For this review, take the finished solid that the model builds, in its own axes (mm). Face numbers are marked on the shaded views. A direction names the side the tool comes from. Round coordinates to 2 decimals unless told otherwise and drop trailing zeros. Loops run counter-clockwise (first coordinate to the right, second up) from the corner with the lowest first, then second, coordinate; pieces in that order, holes last. Notation, with made-up numbers: (75.25, 89.5) -> (132.25, 89.5) arc R17 ccw to (132.25, 99.5) -> close; hole circle Ø10 at (44, 28). An arc over 180 degrees is marked (long way). One line per question, with ' | ' between items. Start each with the question number.
1. Consider section D-D (x = 7). Write out the cut boundary in (y, z), and give its area (3 significant figures).
2. For the marked faces 4 and 5, list the 3-axis set-ups (+Z, -Z, +X, -X, +Y, -Y) from which the entire face can be reached by the end or side of a thin tool; tool diameter is ignored.
3. Consider section A-A (z = 0). Write out the cut boundary in (x, y), and give its area (3 significant figures).
4. Draft analysis for pull direction X (two halves, no side actions). For the marked faces 1, 2 and 3, state which applies: pulls with the +X half, pulls with the -X half, needs draft (parallel to the pull), parting line crosses it, or undercut.
5. Wall thickness on line 1 along Y through (x, z) = (14.5, -1.5); line 2 along Y through (x, z) = (12.5, 0); line 3 along X through (y, z) = (41, 0): over which ranges is each line inside the solid? List them lowest first.
6. For pin 1 Ø2 at (x, y) = (-0.5, 20) entering from -Z; pin 2 Ø10 at (x, y) = (-3, 26.5) entering from +Z; pin 3 Ø1.5 at (x, z) = (-3, -0.5) entering from +Y; pin 4 Ø8 at (y, z) = (12, 12) entering from -X, all flat-tipped, find the tip position at first contact; note any pin that passes through.
7. Consider section B-B (x = 0). Write out the cut boundary in (y, z), and give its area (4 significant figures).
8. Consider section C-C (y = 51). Write out the cut boundary in (x, z).
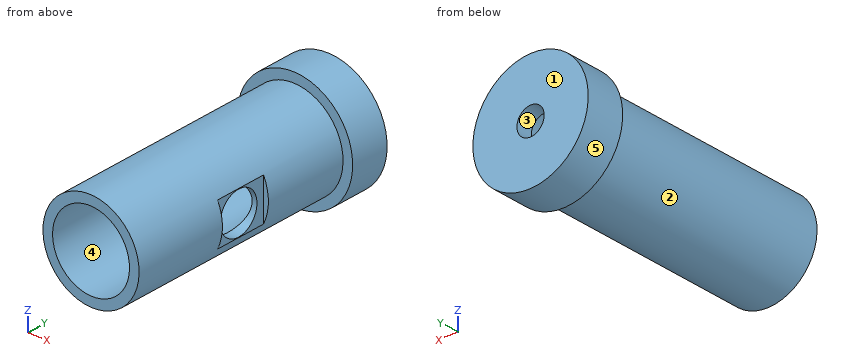
```python
from build123d import *

# Parameters (mm, degrees)
TAGLIO_ESTRUSIONE1_START = 15
SCHIZZO2_W               = 16
SCHIZZO2_H               = 16
TAGLIO_ESTRUSIONE1_DEPTH = 1.5
FORO_12_8_12_8_1_D       = 12.8
FORO_12_8_12_8_1_DEPTH   = 15.154492038
FORO_12_8_12_8_1_TIP     = 3.845507962


with BuildPart() as part:
    # Schizzo1 → Rivoluzione1 (revolve)
    with BuildSketch(Plane.XY, mode=Mode.PRIVATE) as rivoluzione1_sk:
        Polygon((-12, 0), (-15, 0), (-15, 71), (-18, 71), (-18, 83), (-4.25, 83), (-4.25, 78), (-12, 78), align=None)
    revolve(rivoluzione1_sk.sketch.rotate(Axis((0, 0, 0), (0, 1, 0)), 270), axis=Axis((0, 0, 0), (0, 1, 0)))

    # Schizzo2 → Taglio-Estrusione1 (cut)
    with BuildSketch(Plane(origin=(0, 0, 0), x_dir=(0, 0, -1), z_dir=(1, 0, 0)).offset(TAGLIO_ESTRUSIONE1_START)):
        with Locations((0, 37)):
            Rectangle(SCHIZZO2_W, SCHIZZO2_H)
    extrude(amount=-TAGLIO_ESTRUSIONE1_DEPTH, mode=Mode.SUBTRACT)

    # Foro Ø12.8 (12.8)-1
    with Locations(Plane(origin=(13.5, 0, 0), x_dir=(0, 0, -1), z_dir=(1, 0, 0))):
        with Locations((0, 36.304872912)):
            Hole(FORO_12_8_12_8_1_D / 2, depth=FORO_12_8_12_8_1_DEPTH)
            with Locations((0, 0, -(FORO_12_8_12_8_1_DEPTH + FORO_12_8_12_8_1_TIP / 2))):  # 118° drill point
                Cone(0, FORO_12_8_12_8_1_D / 2, FORO_12_8_12_8_1_TIP, mode=Mode.SUBTRACT)


solid = part.part
```
Answer block:
1) outline: (0, -13.27) -> (71, -13.27) -> (71, -16.58) -> (83, -16.58) -> (83, 16.58) -> (71, 16.58) -> (71, 13.27) -> (0, 13.27) -> (0, 9.75) -> (78, 9.75) -> (78, -9.75) -> (0, -9.75) -> close | area: 761 mm2
2) face 4: -Y | face 5: +Y, -Y
3) outline: (-18, 71) -> (-15, 71) -> (-15, 0) -> (-12, 0) -> (-12, 78) -> (-4.25, 78) -> (-4.25, 83) -> (-18, 83) -> close; (4.25, 78) -> (12, 78) -> (12, 42.7) -> (13.5, 42.7) -> (13.5, 45) -> (15, 45) -> (15, 71) -> (18, 71) -> (18, 83) -> (4.25, 83) -> close; (12, 0) -> (15, 0) -> (15, 29) -> (13.5, 29) -> (13.5, 29.9) -> (12, 29.9) -> close | area: 604 mm2
4) face 1: needs draft | face 2: parting line crosses it | face 3: undercut
5) line 1: y = 0 to 29, 45 to 83 | line 2: y = 0 to 29.9, 42.7 to 83 | line 3: x = -15 to -12
6) pin 1: stops at z = -15 | pin 2: stops at z = 15 | pin 3: passes through | pin 4: stops at x = -12.69
7) outline: (0, -15) -> (71, -15) -> (71, -18) -> (83, -18) -> (83, -4.25) -> (78, -4.25) -> (78, -12) -> (0, -12) -> close; (0, 12) -> (78, 12) -> (78, 4.25) -> (83, 4.25) -> (83, 18) -> (71, 18) -> (71, 15) -> (0, 15) -> close | area: 647.5 mm2
8) outline: circle Ø30 at (0, 0); hole circle Ø24 at (0, 0)
